```python
from build123d import *

# Parameters (mm, degrees)
SKETCH1_W               = 72
SKETCH1_H               = 40
BOSS_EXTRUDE1_DEPTH     = 26
BOSS_EXTRUDE3_START     = -5
SKETCH1_4_R             = 9
SKETCH1_4_R_2           = 4
BOSS_EXTRUDE3_DEPTH     = 34
CUT_EXTRUDE2_DEPTH      = 177.028406798
CUT_EXTRUDE2_DEPTH_BACK = 177.028406798
CUT_EXTRUDE3_DEPTH      = 177.028406798
CUT_EXTRUDE3_DEPTH_BACK = 177.028406798
SKETCH3_R               = 2.5
FILLET1_R               = 5


with BuildPart() as part:
    # Sketch1 → Boss-Extrude1 (new body)
    # profile 1 of 2: a face of its own
    with BuildSketch(Plane.XY):
        with BuildLine():
            Line((87, 88), (33, 88))
            ThreePointArc((33, 88), (24, 79), (15, 88))
            Line((15, 88), (12, 88))
            ThreePointArc((12, 88), (3.514718626, 84.485281374), (0, 76))
            Line((0, 76), (0, 12))
            ThreePointArc((0, 12), (3.514718626, 3.514718626), (12, 0))
            Line((12, 0), (15, 0))
            ThreePointArc((15, 0), (24, 9), (33, 0))
            Line((33, 0), (87, 0))
            ThreePointArc((87, 0), (96, 9), (105, 0))
            Line((105, 0), (132, 0))
            ThreePointArc((132, 0), (140.485281374, 3.514718626), (144, 12))
            Line((144, 12), (144, 76))
            ThreePointArc((144, 76), (140.485281374, 84.485281374), (132, 88))
            Line((132, 88), (105, 88))
            ThreePointArc((105, 88), (96, 79), (87, 88))
        make_face()
        with Locations((72, 44)):
            Rectangle(SKETCH1_W, SKETCH1_H, mode=Mode.SUBTRACT)
    # profile 2 of 2: a face of its own
    with BuildSketch(Plane.XY):
        with Locations((72, 44)):
            Rectangle(SKETCH1_W, SKETCH1_H)
    extrude(amount=BOSS_EXTRUDE1_DEPTH)

    # Sketch1<4> → Boss-Extrude3 (add)
    # profile 1 of 4: a face of its own
    with BuildSketch(Plane.XY.offset(BOSS_EXTRUDE3_START)):
        with Locations((24, 88)):
            Circle(SKETCH1_4_R)
        with Locations((24, 88)):
            Circle(SKETCH1_4_R_2, mode=Mode.SUBTRACT)
    # profile 2 of 4: a face of its own
    with BuildSketch(Plane.XY.offset(BOSS_EXTRUDE3_START)):
        with Locations((96, 88)):
            Circle(SKETCH1_4_R)
        with Locations((96, 88)):
            Circle(SKETCH1_4_R_2, mode=Mode.SUBTRACT)
    # profile 3 of 4: a face of its own
    with BuildSketch(Plane.XY.offset(BOSS_EXTRUDE3_START)):
        with Locations((96, 0)):
            Circle(SKETCH1_4_R)
        with Locations((96, 0)):
            Circle(SKETCH1_4_R_2, mode=Mode.SUBTRACT)
    # profile 4 of 4: a face of its own
    with BuildSketch(Plane.XY.offset(BOSS_EXTRUDE3_START)):
        with Locations((24, 0)):
            Circle(SKETCH1_4_R)
        with Locations((24, 0)):
            Circle(SKETCH1_4_R_2, mode=Mode.SUBTRACT)
    extrude(amount=BOSS_EXTRUDE3_DEPTH)

    # Sketch2 → Cut-Extrude2 (cut, two sides: drawn at the far end of the back side and taken through both)
    with BuildSketch(Plane(origin=(0, 0, 0), x_dir=(0, 0, -1), z_dir=(1, 0, 0)).offset(-CUT_EXTRUDE2_DEPTH_BACK)):
        with BuildLine():
            Line((-13, 25), (-13, 63))
            ThreePointArc((-13, 63), (-13.878679656, 65.121320344), (-16, 66))
            Line((-16, 66), (-26, 66))
            Line((-26, 66), (-26, 22))
            Line((-26, 22), (-16, 22))
            ThreePointArc((-16, 22), (-13.878679656, 22.878679656), (-13, 25))
        make_face()
    extrude(amount=CUT_EXTRUDE2_DEPTH + CUT_EXTRUDE2_DEPTH_BACK, mode=Mode.SUBTRACT)

    # Sketch3 → Cut-Extrude3 (cut, two sides: drawn at the far end of the back side and taken through both)
    with BuildSketch(Plane(origin=(0, 0, 0), x_dir=(1, 0, 0), z_dir=(0, 1, 0)).offset(-CUT_EXTRUDE3_DEPTH_BACK)):
        with Locations(Location((113, -21, 0), (0, 0, 270))):
            Circle(SKETCH3_R)
        with Locations(Location((123, -21, 0), (0, 0, 270))):
            Circle(SKETCH3_R)
        with BuildLine():
            Line((72, -17.333333333), (48, -17.333333333))
            ThreePointArc((48, -17.333333333), (45.878679656, -18.21201299), (45, -20.333333333))
            Line((45, -20.333333333), (45, -26))
            Line((45, -26), (75, -26))
            Line((75, -26), (75, -20.333333333))
            ThreePointArc((75, -20.333333333), (74.121320344, -18.21201299), (72, -17.333333333))
        make_face()
    extrude(amount=CUT_EXTRUDE3_DEPTH + CUT_EXTRUDE3_DEPTH_BACK, mode=Mode.SUBTRACT)

    # Fillet1
    # the kernel refuses this fillet: 5 mm, written as the material it takes off along each edge
    with BuildSketch(Plane(origin=(27.5, 88, 0), x_dir=(0, -1, 0), z_dir=(-1, 0, 0))) as fillet1_piece_1_section:
        with BuildLine():
            CenterArc((FILLET1_R, FILLET1_R), FILLET1_R, 180, 90)
            Line((0, FILLET1_R), (0, 0))
            Line((0, 0), (FILLET1_R, 0))
        make_face()
    fillet1_piece_1 = extrude(amount=15.5, mode=Mode.PRIVATE)
    fillet1_piece_1 = fillet1_piece_1 - Plane(origin=(24, 88, 2.038539575), x_dir=(1, 0, 0), z_dir=(0, 0, -1)) * Cylinder(9, 51, mode=Mode.PRIVATE)
    add(fillet1_piece_1, mode=Mode.SUBTRACT)
    with BuildSketch(Plane(origin=(99.5, 88, 0), x_dir=(0, -1, 0), z_dir=(-1, 0, 0))) as fillet1_piece_2_section:
        with BuildLine():
            CenterArc((FILLET1_R, FILLET1_R), FILLET1_R, 180, 90)
            Line((0, FILLET1_R), (0, 0))
            Line((0, 0), (FILLET1_R, 0))
        make_face()
    fillet1_piece_2 = extrude(amount=79, mode=Mode.PRIVATE)
    fillet1_piece_2 = fillet1_piece_2 - Plane(origin=(24, 88, 1.113779656), x_dir=(1, 0, 0), z_dir=(0, 0, -1)) * Cylinder(9, 178, mode=Mode.PRIVATE)
    fillet1_piece_2 = fillet1_piece_2 - Plane(origin=(96, 88, 1.113779656), x_dir=(1, 0, 0), z_dir=(0, 0, -1)) * Cylinder(9, 178, mode=Mode.PRIVATE)
    add(fillet1_piece_2, mode=Mode.SUBTRACT)
    with BuildSketch(Plane(origin=(132, 88, 0), x_dir=(0, -1, 0), z_dir=(-1, 0, 0))) as fillet1_piece_3_section:
        with BuildLine():
            CenterArc((FILLET1_R, FILLET1_R), FILLET1_R, 180, 90)
            Line((0, FILLET1_R), (0, 0))
            Line((0, 0), (FILLET1_R, 0))
        make_face()
    fillet1_piece_3 = extrude(amount=39.5, mode=Mode.PRIVATE)
    fillet1_piece_3 = fillet1_piece_3 - Plane(origin=(96, 88, 0.84758794), x_dir=(1, 0, 0), z_dir=(0, 0, -1)) * Cylinder(9, 99, mode=Mode.PRIVATE)
    add(fillet1_piece_3, mode=Mode.SUBTRACT)
    with BuildSketch(Plane(origin=(132, 76, 0), x_dir=(1, 0, 0), z_dir=(0, -1, 0))) as fillet1_piece_4:
        with BuildLine():
            CenterArc((12 - FILLET1_R, FILLET1_R), FILLET1_R, 270, 90)
            Line((12, FILLET1_R), (12, 0))
            Line((12, 0), (12 - FILLET1_R, 0))
        make_face()
    revolve(axis=Axis((132, 76, 0), (0, 0, 1)), revolution_arc=90, mode=Mode.SUBTRACT)
    with BuildSketch(Plane(origin=(144, 12, 0), x_dir=(-1, 0, 0), z_dir=(0, 1, 0)), Plane(origin=(0, 76, 0), x_dir=(1, 0, 0), z_dir=(0, -1, 0))) as fillet1_piece_5:
        with BuildLine():
            CenterArc((FILLET1_R, FILLET1_R), FILLET1_R, 180, 90)
            Line((0, FILLET1_R), (0, 0))
            Line((0, 0), (FILLET1_R, 0))
        make_face()
    extrude(amount=64, mode=Mode.SUBTRACT)
    with BuildSketch(Plane(origin=(132, 12, 0), x_dir=(0, -1, 0), z_dir=(-1, 0, 0))) as fillet1_piece_6:
        with BuildLine():
            CenterArc((12 - FILLET1_R, FILLET1_R), FILLET1_R, 270, 90)
            Line((12, FILLET1_R), (12, 0))
            Line((12, 0), (12 - FILLET1_R, 0))
        make_face()
    revolve(axis=Axis((132, 12, 0), (0, 0, 1)), revolution_arc=90, mode=Mode.SUBTRACT)
    with BuildSketch(Plane(origin=(92.5, 0, 0), x_dir=(0, 1, 0), z_dir=(1, 0, 0))) as fillet1_piece_7_section:
        with BuildLine():
            CenterArc((FILLET1_R, FILLET1_R), FILLET1_R, 180, 90)
            Line((0, FILLET1_R), (0, 0))
            Line((0, 0), (FILLET1_R, 0))
        make_face()
    fillet1_piece_7 = extrude(amount=39.5, mode=Mode.PRIVATE)
    fillet1_piece_7 = fillet1_piece_7 - Plane(origin=(96, 0, 1.166964438), x_dir=(1, 0, 0), z_dir=(0, 0, -1)) * Cylinder(9, 99, mode=Mode.PRIVATE)
    add(fillet1_piece_7, mode=Mode.SUBTRACT)
    with BuildSketch(Plane(origin=(20.5, 0, 0), x_dir=(0, 1, 0), z_dir=(1, 0, 0))) as fillet1_piece_8_section:
        with BuildLine():
            CenterArc((FILLET1_R, FILLET1_R), FILLET1_R, 180, 90)
            Line((0, FILLET1_R), (0, 0))
            Line((0, 0), (FILLET1_R, 0))
        make_face()
    fillet1_piece_8 = extrude(amount=79, mode=Mode.PRIVATE)
    fillet1_piece_8 = fillet1_piece_8 - Plane(origin=(96, 0, 1.113779656), x_dir=(1, 0, 0), z_dir=(0, 0, -1)) * Cylinder(9, 178, mode=Mode.PRIVATE)
    fillet1_piece_8 = fillet1_piece_8 - Plane(origin=(24, 0, 1.113779656), x_dir=(1, 0, 0), z_dir=(0, 0, -1)) * Cylinder(9, 178, mode=Mode.PRIVATE)
    add(fillet1_piece_8, mode=Mode.SUBTRACT)
    with BuildSketch(Plane(origin=(12, 0, 0), x_dir=(0, 1, 0), z_dir=(1, 0, 0))) as fillet1_piece_9_section:
        with BuildLine():
            CenterArc((FILLET1_R, FILLET1_R), FILLET1_R, 180, 90)
            Line((0, FILLET1_R), (0, 0))
            Line((0, 0), (FILLET1_R, 0))
        make_face()
    fillet1_piece_9 = extrude(amount=15.5, mode=Mode.PRIVATE)
    fillet1_piece_9 = fillet1_piece_9 - Plane(origin=(24, 0, 0.994853316), x_dir=(1, 0, 0), z_dir=(0, 0, -1)) * Cylinder(9, 51, mode=Mode.PRIVATE)
    add(fillet1_piece_9, mode=Mode.SUBTRACT)
    with BuildSketch(Plane(origin=(12, 12, 0), x_dir=(-1, 0, 0), z_dir=(0, 1, 0))) as fillet1_piece_10:
        with BuildLine():
            CenterArc((12 - FILLET1_R, FILLET1_R), FILLET1_R, 270, 90)
            Line((12, FILLET1_R), (12, 0))
            Line((12, 0), (12 - FILLET1_R, 0))
        make_face()
    revolve(axis=Axis((12, 12, 0), (0, 0, 1)), revolution_arc=90, mode=Mode.SUBTRACT)
    with BuildSketch(Plane(origin=(12, 76, 0), x_dir=(0, 1, 0), z_dir=(1, 0, 0))) as fillet1_piece_11:
        with BuildLine():
            CenterArc((12 - FILLET1_R, FILLET1_R), FILLET1_R, 270, 90)
            Line((12, FILLET1_R), (12, 0))
            Line((12, 0), (12 - FILLET1_R, 0))
        make_face()
    revolve(axis=Axis((12, 76, 0), (0, 0, 1)), revolution_arc=90, mode=Mode.SUBTRACT)


solid = part.part
```
The listing builds one solid part. Answer for the finished solid, in the listing's coordinates (mm). A direction names the side the tool comes from. Give positions to 0.01 mm unless a question says otherwise; leave off trailing zeros. Order: outer loops, then holes, each group sorted by start corner. A loop starts at its lowest first (then second) coordinate and runs counter-clockwise, first axis right, second up.
1) Find section C-C on z = 8. Write down the section's boundary in (x, y).
Reported:
outline: (0, 12) arc R12 ccw to (12, 0) - (15, 0) arc R9 ccw to (33, 0) - (87, 0) arc R9 ccw to (105, 0) - (132, 0) arc R12 ccw to (144, 12) - (144, 76) arc R12 ccw to (132, 88) - (105, 88) arc R9 ccw to (87, 88) - (33, 88) arc R9 ccw to (15, 88) - (12, 88) arc R12 ccw to (0, 76) - close; hole circle Ø8 at (24, 0); hole circle Ø8 at (24, 88); hole circle Ø8 at (96, 0); hole circle Ø8 at (96, 88)
2) Consider line 1 along Y through (x, z) = (24, 10); line 2 along X through (y, z) = (11.75, 21); line 3 along Z through (x, y) = (113, 10). Determine where each line is inside the solid, lowest interval first.
Reported:
line 1: y = -9 to -4, 4 to 84, 92 to 97
line 2: x = 0 to 45, 75 to 110.5, 115.5 to 120.5, 125.5 to 144
line 3: z = 0 to 18.5, 23.5 to 26
3) Find section B-B on x = 24. Write down the section's boundary in (y, z), then the cut area to 3 significant figures.
Reported:
outline: (-9, -5) - (-4, -5) - (-4, 29) - (-9, 29) - close; (4, -5) - (9, -5) - (9, 0) - (79, 0) - (79, -5) - (84, -5) - (84, 29) - (79, 29) - (79, 26) - (66, 26) - (66, 16) arc R3 cw to (63, 13) - (25, 13) arc R3 cw to (22, 16) - (22, 26) - (9, 26) - (9, 29) - (4, 29) - close; (92, -5) - (97, -5) - (97, 29) - (92, 29) - close
area: 1,930 mm2
4) For faces 1 (the face through (60, 0, 13)), 2 (the face through (22, 75, 26)), 3 (the face through (45, 11, 23)), 4 (the face through (70.99, 65.1, 13.86)), determine the directions among +Z, -Z, +X, -X, +Y, -Y from which every point of the face is accessible in a straight line to the end or side of a thin tool.
Reported:
face 1: +Z, -Z, -Y
face 2: +Z
face 3: +Z, +Y, -Y
face 4: +Z, +X, -X
5) Find section A-A on y = 70. Write down the section's boundary in (x, z), then the cut area to 3 significant figures.
Reported:
outline: (0, 5) arc R5 ccw to (5, 0) - (139, 0) arc R5 ccw to (144, 5) - (144, 26) - (75, 26) - (75, 20.33) arc R3 cw to (72, 17.33) - (48, 17.33) arc R3 cw to (45, 20.33) - (45, 26) - (0, 26) - close; hole circle Ø5 at (113, 21); hole circle Ø5 at (123, 21)
area: 3,440 mm2
6) Given P1, Ø10, axis at x = 31.5, z = 23.5, coming from the +Y side; P2, Ø0.9, axis at x = 14, z = 18, coming from the -Y side; P3, Ø17.5, axis at x = 12, y = 74, coming from the +Z side; P4, Ø5, axis at x = 24, y = 88, coming from the +Z side, each flat-ended and moving along its own axis, determine where each tip first touches the part or whether it passes through.
Reported:
P1: stops at y = 96.65
P2: stops at y = 0
P3: stops at z = 26
P4: passes through
7) Determine the mould class of faces 5 (the face through (60, 77, 17.333)), 6 (the face through (14, 88, 15)), 7 (the face through (92, 0, 12)) for opening direction Y: pulls with the +Y half, pulls with the -Y half, needs draft (parallel to the pull), parting line crosses it, or undercut.
Reported:
face 5: needs draft
face 6: pulls with the +Y half
face 7: undercut
8) Find section D-D on x = 78.5. Write down the section's boundary in (y, z), then the cut area to 3 significant figures.
Reported:
outline: (0, 5) arc R5 ccw to (5, 0) - (83, 0) arc R5 ccw to (88, 5) - (88, 26) - (66, 26) - (66, 16) arc R3 cw to (63, 13) - (25, 13) arc R3 cw to (22, 16) - (22, 26) - (0, 26) - close
area: 1,710 mm2
